Could you check a few things on this model? Use its own coordinates, in mm. A direction names the side the tool comes from. Coordinates: 2 decimals unless noted, no trailing zeros. Write each loop counter-clockwise with the first axis right and the second up, starting at its lowest first coordinate (ties: lowest second). Pieces come first, ordered by that corner, then holes.
Item 1: For P1, Ø1, axis at x = -2.5, y = 1, coming from the -Z side; P2, Ø0.9, axis at x = 3.5, z = 1.5, coming from the +Y side; P3, Ø0.9, axis at x = -3.5, z = 1, coming from the -Y side; P4, Ø1, axis at y = 31.5, z = 2, coming from the +X side, each with a flat end and sliding along its axis, tell me the tip position at first contact or that it passes through.
Item 2: I want a section at B-B on x = 4.5. Please give me the cut outline in (y, z) (3 decimals), then the cut area to 3 significant figures.
Item 3: If I drill on probe 1 along Y at (x, z) = (-2.75, 2.9), over which ranges is the centre line in solid material (lowest first)?
Item 4: Which directions (+Z, -Z, +X, -X, +Y, -Y) give clear straight access to the entire face, cutting with the end or side of a thin tool? Please do faces 1 (the flat face through (-2.041, 32, 2)), 2 (the flat face through (4, 30.041, 2)), 3 (the flat face through (-5.041, 0, 2)), 4 (the flat face through (2.041, -32, 2)), 5 (the flat face through (-4, -30.041, 2)).
Item 5: I want a section at A-A on z = 1.6. Please give me the cut outline in (x, y).
from build123d import *

# Parameters (mm, degrees)
SKETCH1_W           = 10
SKETCH1_H           = 60
SKETCH1_W_2         = 4
SKETCH1_H_2         = 3.175
BOSS_EXTRUDE1_DEPTH = 3.175
BOSS_EXTRUDE2_DEPTH = 3.175


with BuildPart() as part:
    # Sketch1 → Boss-Extrude1 (new body)
    with BuildSketch(Plane.XY):
        Rectangle(SKETCH1_W, SKETCH1_H)
        with Locations((0, 31.5875)):
            Rectangle(SKETCH1_W_2, SKETCH1_H_2)
        with Locations((0, -31.5875)):
            Rectangle(SKETCH1_W_2, SKETCH1_H_2)
    extrude(amount=BOSS_EXTRUDE1_DEPTH)

    # Sketch2 → Boss-Extrude2 (add)
    with BuildSketch(Plane.XY.offset(3.175)):
        Polygon((5.04064, -30.04064), (5.04064, 30.04064), (2.04064, 30.04064), (2.04064, 33.21564), (-2.04064, 33.21564), (-2.04064, 30.04064), (-5.04064, 30.04064), (-5.04064, -30.04064), (-2.04064, -30.04064), (-2.04064, -33.21564), (2.04064, -33.21564), (2.04064, -30.04064), align=None)
    extrude(amount=-BOSS_EXTRUDE2_DEPTH)


solid = part.part
Response values:
1. P1: stops at z = 0
1. P2: stops at y = 30.04
1. P3: stops at y = -30.04
1. P4: stops at x = 2.04
2. outline: (-30.041, 0) - (30.041, 0) - (30.041, 3.175) - (-30.041, 3.175) - close
2. area: 191 mm2
3. probe 1: y = -30.04 to 30.04
4. face 1: +Z, -Z, -X, +Y
4. face 2: +Z, -Z, +X, +Y
4. face 3: +Z, -Z, -X, +Y, -Y
4. face 4: +Z, -Z, +X, -Y
4. face 5: +Z, -Z, -X, -Y
5. outline: (-5.04, -30.04) - (-2.04, -30.04) - (-2.04, -33.22) - (2.04, -33.22) - (2.04, -30.04) - (5.04, -30.04) - (5.04, 30.04) - (2.04, 30.04) - (2.04, 33.22) - (-2.04, 33.22) - (-2.04, 30.04) - (-5.04, 30.04) - close
